```python
from build123d import *

# Parameters (mm, degrees)
SKETCH1_R           = 60
SKETCH1_R_2         = 3
SKETCH1_R_3         = 2.75
BOSS_EXTRUDE1_DEPTH = 3


with BuildPart() as part:
    # Sketch1 → Boss-Extrude1 (new body)
    with BuildSketch(Plane.XY):
        Circle(SKETCH1_R)
        with Locations((0, 20)):
            Circle(SKETCH1_R_2, mode=Mode.SUBTRACT)
        with Locations((17.320508076, -10)):
            Circle(SKETCH1_R_2, mode=Mode.SUBTRACT)
        with Locations((-17.320508076, -10)):
            Circle(SKETCH1_R_2, mode=Mode.SUBTRACT)
        with Locations((0, 53.710768159)):
            Circle(SKETCH1_R_3, mode=Mode.SUBTRACT)
        with Locations((8.203059397, 48.487448679)):
            Circle(SKETCH1_R_3, mode=Mode.SUBTRACT)
        with Locations((24.29203853, 42.757686174)):
            Circle(SKETCH1_R_3, mode=Mode.SUBTRACT)
        with Locations((18.370164624, 50.471612496)):
            Circle(SKETCH1_R_3, mode=Mode.SUBTRACT)
        with Locations((37.451039304, 31.87071568)):
            Circle(SKETCH1_R_3, mode=Mode.SUBTRACT)
        with Locations((34.524616279, 41.144835484)):
            Circle(SKETCH1_R_3, mode=Mode.SUBTRACT)
        with Locations((46.09289202, 17.139666513)):
            Circle(SKETCH1_R_3, mode=Mode.SUBTRACT)
        with Locations((46.514889682, 26.855384079)):
            Circle(SKETCH1_R_3, mode=Mode.SUBTRACT)
        with Locations((49.175261699, 0.34132061)):
            Circle(SKETCH1_R_3, mode=Mode.SUBTRACT)
        with Locations((52.894780903, 9.326777012)):
            Circle(SKETCH1_R_3, mode=Mode.SUBTRACT)
        with Locations((46.326369068, -16.498193596)):
            Circle(SKETCH1_R_3, mode=Mode.SUBTRACT)
        with Locations((52.894780903, -9.326777012)):
            Circle(SKETCH1_R_3, mode=Mode.SUBTRACT)
        with Locations((37.889832623, -31.347782166)):
            Circle(SKETCH1_R_3, mode=Mode.SUBTRACT)
        with Locations((46.514889682, -26.855384079)):
            Circle(SKETCH1_R_3, mode=Mode.SUBTRACT)
        with Locations((24.883223169, -42.416365564)):
            Circle(SKETCH1_R_3, mode=Mode.SUBTRACT)
        with Locations((34.524616279, -41.144835484)):
            Circle(SKETCH1_R_3, mode=Mode.SUBTRACT)
        with Locations((8.875329764, -48.368909275)):
            Circle(SKETCH1_R_3, mode=Mode.SUBTRACT)
        with Locations((18.370164624, -50.471612496)):
            Circle(SKETCH1_R_3, mode=Mode.SUBTRACT)
        with Locations((-8.203059397, -48.487448679)):
            Circle(SKETCH1_R_3, mode=Mode.SUBTRACT)
        with Locations((0, -53.710768159)):
            Circle(SKETCH1_R_3, mode=Mode.SUBTRACT)
        with Locations((-24.29203853, -42.757686174)):
            Circle(SKETCH1_R_3, mode=Mode.SUBTRACT)
        with Locations((-18.370164624, -50.471612496)):
            Circle(SKETCH1_R_3, mode=Mode.SUBTRACT)
        with Locations((-37.451039304, -31.87071568)):
            Circle(SKETCH1_R_3, mode=Mode.SUBTRACT)
        with Locations((-34.524616279, -41.144835484)):
            Circle(SKETCH1_R_3, mode=Mode.SUBTRACT)
        with Locations((-46.09289202, -17.139666513)):
            Circle(SKETCH1_R_3, mode=Mode.SUBTRACT)
        with Locations((-46.514889682, -26.855384079)):
            Circle(SKETCH1_R_3, mode=Mode.SUBTRACT)
        with Locations((-49.175261699, -0.34132061)):
            Circle(SKETCH1_R_3, mode=Mode.SUBTRACT)
        with Locations((-52.894780903, -9.326777012)):
            Circle(SKETCH1_R_3, mode=Mode.SUBTRACT)
        with Locations((-46.326369068, 16.498193596)):
            Circle(SKETCH1_R_3, mode=Mode.SUBTRACT)
        with Locations((-52.894780903, 9.326777012)):
            Circle(SKETCH1_R_3, mode=Mode.SUBTRACT)
        with Locations((-37.889832623, 31.347782166)):
            Circle(SKETCH1_R_3, mode=Mode.SUBTRACT)
        with Locations((-46.514889682, 26.855384079)):
            Circle(SKETCH1_R_3, mode=Mode.SUBTRACT)
        with Locations((-24.883223169, 42.416365564)):
            Circle(SKETCH1_R_3, mode=Mode.SUBTRACT)
        with Locations((-34.524616279, 41.144835484)):
            Circle(SKETCH1_R_3, mode=Mode.SUBTRACT)
        with Locations((-8.875329764, 48.368909275)):
            Circle(SKETCH1_R_3, mode=Mode.SUBTRACT)
        with Locations((-18.370164624, 50.471612496)):
            Circle(SKETCH1_R_3, mode=Mode.SUBTRACT)
        with BuildLine():
            Line((-3.577708764, 3.2), (3.577708764, 3.2))
            ThreePointArc((3.577708764, 3.2), (0, -4.8), (-3.577708764, 3.2))
        make_face(mode=Mode.SUBTRACT)
        with BuildLine():
            ThreePointArc((-36.685477237, 22.431579524), (-41.887860306, 9.716334647), (-42.814413921, -3.990734342))
            ThreePointArc((-42.814413921, -3.990734342), (-42.633094621, -4.655838122), (-42.236723549, -5.219867997))
            ThreePointArc((-42.236723549, -5.219867997), (-37.395188654, -8.1165077), (-31.759641982, -8.384080905))
            ThreePointArc((-31.759641982, -8.384080905), (-30.36605231, -7.319812925), (-30.346741444, -5.566420328))
            ThreePointArc((-30.346741444, -5.566420328), (-33.974787858, 7.440990576), (-33.036641088, 20.912268907))
            ThreePointArc((-33.036641088, 20.912268907), (-34.210392666, 23.23459047), (-36.685477237, 22.431579524))
        make_face(mode=Mode.SUBTRACT)
        with BuildLine():
            ThreePointArc((-19.994032134, 23.497838848), (-10.543307061, 33.143524662), (1.59223558, 39.066704891))
            ThreePointArc((1.59223558, 39.066704891), (3.01654926, 41.244364357), (1.083579096, 42.986344999))
            ThreePointArc((1.083579096, 42.986344999), (-12.529337517, 41.134118459), (-24.863284281, 35.083002933))
            ThreePointArc((-24.863284281, 35.083002933), (-25.3486214, 34.593423923), (-25.638900064, 33.968141567))
            ThreePointArc((-25.638900064, 33.968141567), (-25.726696185, 28.326929504), (-23.140648042, 23.312616319))
            ThreePointArc((-23.140648042, 23.312616319), (-21.522170099, 22.637866251), (-19.994032134, 23.497838848))
        make_face(mode=Mode.SUBTRACT)
        with BuildLine():
            ThreePointArc((8.61899394, 31.696697224), (11.668492469, 36.443437203), (16.597823485, 39.188009564))
            ThreePointArc((16.597823485, 39.188009564), (17.284473221, 39.249262045), (17.95112964, 39.073737275))
            ThreePointArc((17.95112964, 39.073737275), (29.358522789, 31.417783812), (37.769056333, 20.554765475))
            ThreePointArc((37.769056333, 20.554765475), (37.226941927, 18.009773887), (34.628876668, 18.154435984))
            ThreePointArc((34.628876668, 18.154435984), (23.431480798, 25.702534085), (10.35270931, 29.064259176))
            ThreePointArc((10.35270931, 29.064259176), (8.843882212, 29.957679176), (8.61899394, 31.696697224))
        make_face(mode=Mode.SUBTRACT)
        with BuildLine():
            ThreePointArc((31.759641982, 8.384080905), (37.395188654, 8.1165077), (42.236723549, 5.219867997))
            ThreePointArc((42.236723549, 5.219867997), (42.633094621, 4.655838122), (42.814413921, 3.990734342))
            ThreePointArc((42.814413921, 3.990734342), (41.887860306, -9.716334647), (36.685477237, -22.431579524))
            ThreePointArc((36.685477237, -22.431579524), (34.210392666, -23.23459047), (33.036641088, -20.912268907))
            ThreePointArc((33.036641088, -20.912268907), (33.974787858, -7.440990576), (30.346741444, 5.566420328))
            ThreePointArc((30.346741444, 5.566420328), (30.36605231, 7.319812925), (31.759641982, 8.384080905))
        make_face(mode=Mode.SUBTRACT)
        with BuildLine():
            ThreePointArc((23.140648042, -23.312616319), (25.726696185, -28.326929504), (25.638900064, -33.968141567))
            ThreePointArc((25.638900064, -33.968141567), (25.3486214, -34.593423923), (24.863284281, -35.083002933))
            ThreePointArc((24.863284281, -35.083002933), (12.529337517, -41.134118459), (-1.083579096, -42.986344999))
            ThreePointArc((-1.083579096, -42.986344999), (-3.01654926, -41.244364357), (-1.59223558, -39.066704891))
            ThreePointArc((-1.59223558, -39.066704891), (10.543307061, -33.143524662), (19.994032134, -23.497838848))
            ThreePointArc((19.994032134, -23.497838848), (21.522170099, -22.637866251), (23.140648042, -23.312616319))
        make_face(mode=Mode.SUBTRACT)
        with BuildLine():
            ThreePointArc((-8.61899394, -31.696697224), (-11.668492469, -36.443437203), (-16.597823485, -39.188009564))
            ThreePointArc((-16.597823485, -39.188009564), (-17.284473221, -39.249262045), (-17.95112964, -39.073737275))
            ThreePointArc((-17.95112964, -39.073737275), (-29.358522789, -31.417783812), (-37.769056333, -20.554765475))
            ThreePointArc((-37.769056333, -20.554765475), (-37.226941927, -18.009773887), (-34.628876668, -18.154435984))
            ThreePointArc((-34.628876668, -18.154435984), (-23.431480798, -25.702534085), (-10.35270931, -29.064259176))
            ThreePointArc((-10.35270931, -29.064259176), (-8.843882212, -29.957679176), (-8.61899394, -31.696697224))
        make_face(mode=Mode.SUBTRACT)
    extrude(amount=BOSS_EXTRUDE1_DEPTH)


solid = part.part
```
Input: part model. Units: mm. Frame: model coordinates. Coordinates: 2 decimals unless noted, no trailing zeros.
1) Pin query (flat end, axial travel): pin 1 Ø4.5 at (x, y) = (46.09, 17.14) entering from +Z; pin 2 Ø1.5 at (y, z) = (-45.5, 1) entering from +X; pin 3 Ø6.5 at (x, y) = (0, 53.71) entering from +Z; pin 4 Ø1.5 at (x, z) = (31.5, 0.5) entering from -Y. Return the tip coordinate at first contact, or that it passes through.
2) Mould query, pull axis X, two halves, no side actions, for faces 1 (the cylindrical face through (-59.94, 2.64, 1.48)), 2 (the cylindrical face through (26.83, 41.7, 1.48)). Classes: pulls with the +X half, pulls with the -X half, needs draft (parallel to the pull), parting line crosses it, or undercut.
3) Material intervals for line 1 along Y through (x, z) = (-54, 1.6); line 2 along Y through (x, z) = (-47.5, 2.85); line 3 along X through (y, z) = (-16.5, 2.15), sorted ascending.
4) Section A-A on z = 0.65. State how many separate pieces and enclosed holes the cut face has, and give its area (3 significant figures).
Check result:
1. pin 1: passes through
1. pin 2: stops at x = 39.97
1. pin 3: stops at z = 3
1. pin 4: stops at y = -51.52
2. face 1: parting line crosses it
2. face 2: undercut
3. line 1: y = -26.15 to -11.84, -6.81 to 6.81, 11.84 to 26.15
3. line 2: y = -36.66 to -29.42, -24.29 to -19.5, -14.78 to -2.52, 1.84 to 14.01, 18.99 to 24.29, 29.42 to 36.66
3. line 3: x = -57.69 to -48.77, -43.42 to 33.86, 39.71 to 43.58, 49.08 to 57.69
4. separate pieces: 1
4. enclosed holes: 46
4. area: 8,770 mm2
